The model under review builds one solid part; all positions refer to its coordinate system, in mm. Face numbers are marked on the shaded views. Coordinates: 2 decimals unless noted, no trailing zeros. Loops run counter-clockwise (first coordinate to the right, second up) from the corner with the lowest first, then second, coordinate; pieces in that order, holes last. Notation, with made-up numbers: M 81,65 L 129,65 A27 ccw 129,97 Z; hole C -30.75,36 d8. An arc over 180 degrees is marked long. Use CSV: the item, a comma, the result in double quotes. Start each with the question number.
1. Clearance check with flat-ended pins moving along their axes: P1, Ø2, axis at y = 0, z = 3.5, coming from the +X side; P2, Ø1.5, axis at x = -11.5, z = -14, coming from the +Y side; P3, Ø4, axis at y = -5.5, z = -9, coming from the +X side. State where each tip first meets the part, or that it passes through.
2. Draft analysis for pull direction Y (two halves, no side actions). For the marked faces 1 and 2, state which applies: +Y half, -Y half, draft (parallel to the pull), parting line (faces both ways), or undercut.
3. Add section D-D, the plane z = 21. Write out the cut boundary in (x, y).
4. Add section B-B, the plane y = -14. Write out the cut boundary in (x, z).
5. Add section A-A, the plane x = -7.5. Write out the cut boundary in (y, z), then the cut area to 3 significant figures.
6. For L1, parallel to Y at x = -4.5, z = 2; L2, parallel to X at y = 0.5, z = -6.5; L3, parallel to Y at x = -12, z = -24, list the stretches that pass through material, from the lowest coordinate up.
7. Add section C-C, the plane x = -3.5. Write out the cut boundary in (y, z).
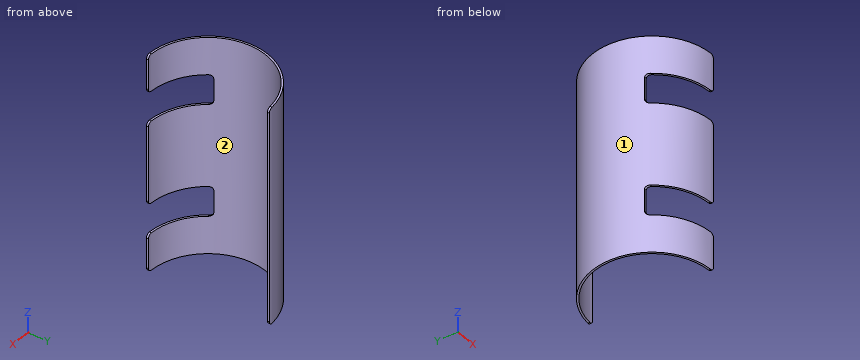
Autodesk Inventor part; units mm, degrees
ref_plane "YZ Plane" through (0, 0, 0) normal (1, 0, 0) x (0, 1, 0)
ref_plane "XZ Plane" through (0, 0, 0) normal (0, 1, 0) x (-1, 0, 0)
ref_plane "XY Plane" through (0, 0, 0) normal (0, 0, 1) x (1, 0, 0)
sketch "Sketch1" plane through (0, 0, 0) normal (0, 0, 1) x (1, 0, 0)
  circle A0 centre (0, 0) radius 15.5
  circle A1 centre (0, 0) radius 16
  dimension "d0" = 32
  dimension "d1" = 0.5
extrude "Extrusion1" add sketch "Sketch1" along normal mid plane 58
sketch "Sketch3" plane through (0, 0, 29) normal (0, 0, 1) x (1, 0, 0)
  circle A0 centre (0, 0) radius 15.5 construction
  circle A1 centre (0, 0) radius 16 construction
  line L0 (0, -20) -> (20, -20)
  line L1 (20, -20) -> (20, 20)
  line L2 (20, 20) -> (0, 20)
  line L3 (0, 20) -> (0, -20)
  dimension "d8" = 20
  dimension "d9" = 40
extrude "Extrusion3" cut sketch "Sketch3" against normal through all
sketch "Sketch4" plane through (0, 0, 0) normal (1, 0, 0) x (0, 1, 0)
  line L0 (-18, -19) -> (-8, -19)
  line L1 (-8, -19) -> (-8, -11)
  line L2 (-8, -11) -> (-18, -11)
  line L3 (-18, -11) -> (-18, -19)
  line L4 (-16, -29) -> (16, -29)
  line L5 (-16, -29) -> (-16, 29)
  point P0 (0, 0)
  dimension "d12" = 8
  dimension "d13" = 10
  dimension "d14" = 2
  dimension "d17" = 8
extrude "Extrusion4" cut sketch "Sketch4" against normal through all
mirror "Mirror1" about plane through (0, 0, 0) normal (0, 0, 1) of "Extrusion4"
fillet "Fillet1" radius 1 12 edges at (0, -15.75, 19) (0, -15.75, 11) (0, -15.75, 29) (0, 15.75, 29) (-13.5662, -8, 19) (-13.5662, -8, 11) (-13.5662, -8, -11) (0, -15.75, -11) (-13.5662, -8, -19) (0, -15.75, -19) (0, -15.75, -29) (0, 15.75, -29)
properties part number "LP-screen-sheet-metal" material "Stainless Steel"
Computed:
1,P1,"stops at x = -15.47"
1,P2,"stops at y = 11.85"
1,P3,"stops at x = -13.56"
2,face 1,"parting line"
2,face 2,"undercut"
3,outline,"M 0,-16 L 0,-15.5 A15.5 cw 0,15.5 L 0,16 A16 ccw Z"
4,outline,"M -7.75,-29 L -6.65,-29 L -6.65,-19 L -7.75,-19 Z; M -7.75,-11 L -6.65,-11 L -6.65,11 L -7.75,11 Z; M -7.75,19 L -6.65,19 L -6.65,29 L -7.75,29 Z"
5,outline,"M -14.13,-29 L -13.56,-29 L -13.56,-19 L -14.13,-19 Z; M -14.13,-11 L -13.56,-11 L -13.56,11 L -14.13,11 Z; M -14.13,19 L -13.56,19 L -13.56,29 L -14.13,29 Z; M 13.56,-29 L 14.13,-29 L 14.13,29 L 13.56,29 Z"
5,area,"56.9 mm^2"
6,L1,"y = -15.35 to -14.83, 14.83 to 15.35"
6,L2,"x = -15.99 to -15.49"
6,L3,"y = -10.58 to -9.81, 9.81 to 10.58"
7,outline,"M -15.61,-29 L -15.1,-29 L -15.1,-19 L -15.61,-19 Z; M -15.61,-11 L -15.1,-11 L -15.1,11 L -15.61,11 Z; M -15.61,19 L -15.1,19 L -15.1,29 L -15.61,29 Z; M 15.1,-29 L 15.61,-29 L 15.61,29 L 15.1,29 Z"
